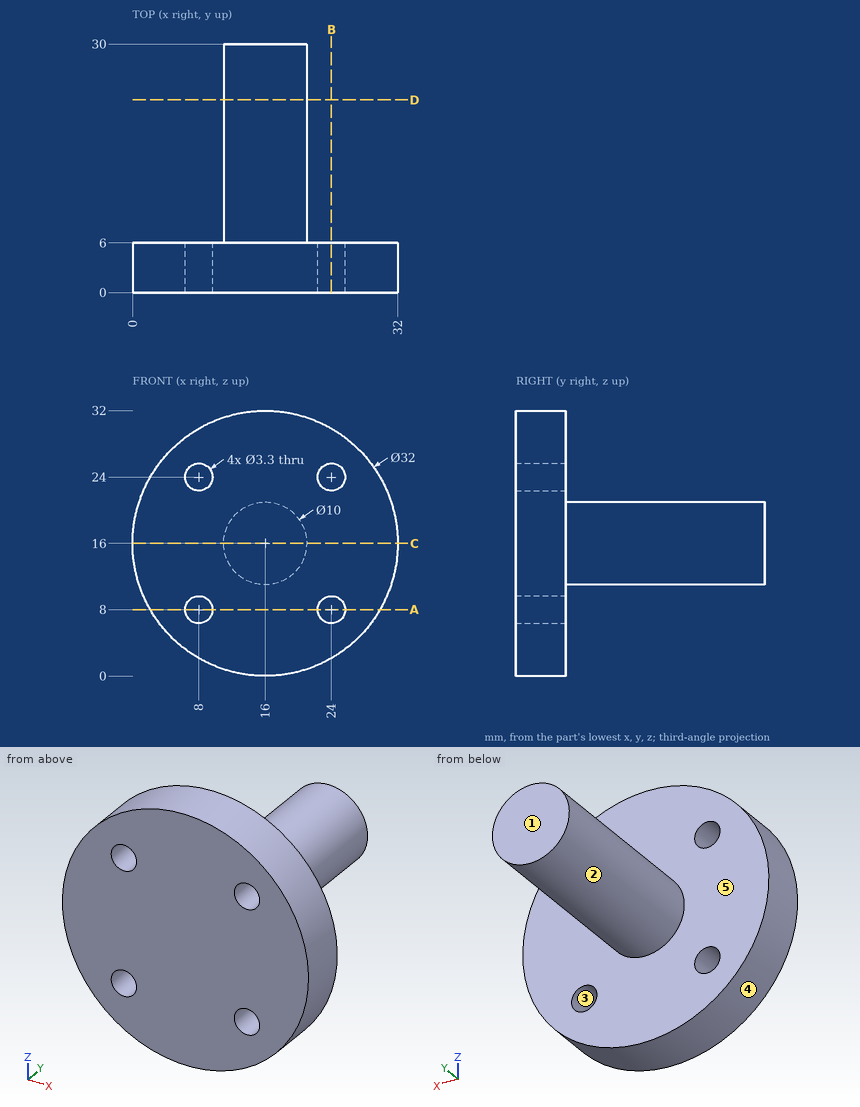
Geometry: see drawing. Coordinates: mm, zero at the bounding-box minimum. A direction names the side the tool comes from. Round coordinates to 2 decimals unless told otherwise and drop trailing zeros. Write each loop counter-clockwise with the first axis right and the second up, starting at its lowest first coordinate (ties: lowest second). Pieces come first, ordered by that corner, then holes. Notation, with made-up numbers: (2.5, 49) -> (40.5, 49) arc R34 cw to (40.5, 87) -> close; hole circle Ø11 at (59, 88.5). An arc over 180 degrees is marked (long way). Answer as CSV lines item,"result".
1. Contact query for flat-ended pins moving along their axis: P1, Ø4, axis at y = 24.5, z = 12.5, coming from the +X side; P2, Ø1, axis at x = 15.5, y = 22.5, coming from the +Z side; P3, Ø4, axis at x = 8, z = 24, coming from the +Y side. Output: stop coordinate, or through.
Geometry says:
P1,"stops at x = 20.77"
P2,"stops at z = 21"
P3,"stops at y = 6"
2. Section A-A (z = 8). Return the cut outline in (x, y), plus the area to 3 significant figures.
Geometry says:
outline,"(2.14, 0) -> (6.35, 0) -> (6.35, 6) -> (2.14, 6) -> close; (9.65, 0) -> (22.35, 0) -> (22.35, 6) -> (9.65, 6) -> close; (25.65, 0) -> (29.86, 0) -> (29.86, 6) -> (25.65, 6) -> close"
area,"127 mm^2"
3. Section B-B (x = 24). Return the cut outline in (y, z).
Geometry says:
outline,"(0, 2.14) -> (6, 2.14) -> (6, 6.35) -> (0, 6.35) -> close; (0, 9.65) -> (6, 9.65) -> (6, 22.35) -> (0, 22.35) -> close; (0, 25.65) -> (6, 25.65) -> (6, 29.86) -> (0, 29.86) -> close"
4. Section D-D (y = 23.25). Return the cut outline in (x, z), plus the area to 3 significant figures.
Geometry says:
outline,"circle Ø10 at (16, 16)"
area,"78.5 mm^2"
5. Reachability of the marked faces 1 and 2 from +Z, -Z, +X, -X, +Y, -Y: full face, straight path, thin tool, end or side. Return the list, or none.
Geometry says:
face 1,"+Z, -Z, +X, -X, +Y"
face 2,"+Y"
6. Ray query, L1, parallel to Z at x = 8, y = 2.05; L2, parallel to Y at x = 14, z = 29.5. Return the intervals inside material, ascending. Write a range as [from, to].
Geometry says:
L1,"z = [2.14, 6.35], [9.65, 22.35], [25.65, 29.86]"
L2,"y = [0, 6]"
7. Section C-C (z = 16). Return the cut outline in (x, y).
Geometry says:
outline,"(0, 0) -> (32, 0) -> (32, 6) -> (21, 6) -> (21, 30) -> (11, 30) -> (11, 6) -> (0, 6) -> close"
8. Mould query, pull axis X, two halves, no side actions, for the marked faces 3, 4 and 5. Classes: +X half, -X half, draft (parallel to the pull), parting line (faces both ways), or undercut.
Geometry says:
face 3,"undercut"
face 4,"parting line"
face 5,"draft"
